from build123d import *

# Parameters (mm, degrees)
F0_W     = 20
F0_H     = 50
F1_DEPTH = 60
F2_R     = 2.5
F3_DEPTH = 20
F4_DEPTH = 40
F5_DEPTH = 40
F6_DEPTH = 25
F7_DEPTH = 40
F8_DEPTH = 15


# Not quite as in the source:
# - a feature names something its author has since deleted; it is built from what else it names


with BuildPart() as f1:
    # F0 (on Top) → F1 (new body)
    with BuildSketch(Plane.XY):
        Rectangle(F0_W, F0_H)
    extrude(amount=F1_DEPTH)

    # F2 (on face) → F3 (cut)
    with BuildSketch(Plane.XZ.offset(25)):
        with Locations((0, 50)):
            Circle(F2_R)
    extrude(amount=-F3_DEPTH, mode=Mode.SUBTRACT)

    # F4 (add): a face of the model
    f4_faces = [f1.faces().sort_by_distance(p)[0] for p in [
        (0, 0, 0),
    ]]
    extrude(f4_faces, amount=-F4_DEPTH)

    # F5 (cut): a face of the model
    f5_faces = [f1.faces().sort_by_distance(p)[0] for p in [
        (0, 0, 0),
    ]]
    extrude(f5_faces, amount=-F5_DEPTH, mode=Mode.SUBTRACT)

    # F6 (cut): a face of the model
    f6_faces = [f1.faces().sort_by_distance(p)[0] for p in [
        (0, 25, 50),
    ]]
    extrude(f6_faces, amount=-F6_DEPTH, mode=Mode.SUBTRACT)

    # F7 (add): a face of the model
    f7_faces = [f1.faces().sort_by_distance(p)[0] for p in [
        (0, -5, 50),
    ]]
    extrude(f7_faces, amount=F7_DEPTH)

    # F8 (cut): a face of the model
    f8_faces = [f1.faces().sort_by_distance(p)[0] for p in [
        (0, 0, 50),
    ]]
    extrude(f8_faces, amount=-F8_DEPTH, mode=Mode.SUBTRACT)


solid = f1.part
Design review of the part built by this model. Coordinates are the model's own, in mm. A direction names the side the tool comes from. Round coordinates to 2 decimals unless told otherwise and drop trailing zeros. Write each loop counter-clockwise with the first axis right and the second up, starting at its lowest first coordinate (ties: lowest second). Pieces come first, ordered by that corner, then holes. Notation, with made-up numbers: (33.5, 36.25) - (89.5, 36.25) arc R25 cw to (89.5, 67.25) - close; hole circle Ø6 at (45.5, 4.25). An arc over 180 degrees is marked (long way). Use a Markdown table: item, result. Add a question column.
1. Wall thickness on probe 1 along Y at (x, z) = (-7.5, 50); probe 2 along Z at (x, y) = (-1.25, -41.75); probe 3 along X at (y, z) = (-35.75, 52.25): over which ranges is each line inside the solid? List them lowest first.
2. We need section B-B (x = 0). State the section outline as (y, z) points.
3. Clearance check with flat-ended pins moving along their axes: pin 1 (12 mm diameter, centred on x = 3.5, y = -27, fed in from +Z); pin 2 (12 mm diameter, centred on x = 2.5, y = -41, fed in from +Z); pin 3 (4 mm diameter, centred on x = 3.5, y = -32.5, fed in from -Z). State where each tip first meets the part, or that it passes through.
4. We need section A-A (z = 50). State the section outline as (x, y) points, then the cut area to 3 significant figures.
5. We need section D-D (z = 46.25). State the section outline as (x, y) points, then the cut area to 3 significant figures.
6. For faces 1 (the face through (0, -15, 50)), 2 (the face through (-0.54, -34.86, 47.56)), list the 3-axis set-ups (+Z, -Z, +X, -X, +Y, -Y) from which the entire face can be reached by the end or side of a thin tool; tool diameter is ignored.
7. We need section C-C (y = -38). State the section outline as (x, z) points.
Output:
| question | item | result |
|---|---|---|
| 1 | probe 1 | y = -25 to -15 |
| 1 | probe 2 | z = 47.83 to 52.17 |
| 1 | probe 3 | x = -1.09 to 1.09 |
| 2 | outline | (-45, 47.5) - (-25, 47.5) - (-25, 40) - (-15, 40) - (-15, 60) - (-25, 60) - (-25, 52.5) - (-45, 52.5) - close |
| 3 | pin 1 | stops at z = 60 |
| 3 | pin 2 | stops at z = 52.5 |
| 3 | pin 3 | stops at z = 48 |
| 4 | outline | (-10, -25) - (-2.5, -25) - (-2.5, -45) - (2.5, -45) - (2.5, -25) - (10, -25) - (10, -15) - (-10, -15) - close |
| 4 | area | 300 mm2 |
| 5 | outline | (-10, -25) - (10, -25) - (10, -15) - (-10, -15) - close |
| 5 | area | 200 mm2 |
| 6 | face 1 | +Z, -Z, +X, -X, +Y |
| 6 | face 2 | -Y |
| 7 | outline | circle Ø5 at (0, 50) |
